The listing builds one solid part. Answer for the finished solid, in the listing's coordinates (mm). Coordinates: 2 decimals unless noted, no trailing zeros. Write each loop counter-clockwise with the first axis right and the second up, starting at its lowest first coordinate (ties: lowest second). Pieces come first, ordered by that corner, then holes. Notation, with made-up numbers: M 3,-12 L 62,-12 A15 cw 62,-6 Z; hole C -25.5,46.5 d7. An arc over 180 degrees is marked long. Put each result on its own line as item: value. Start each with the question number.
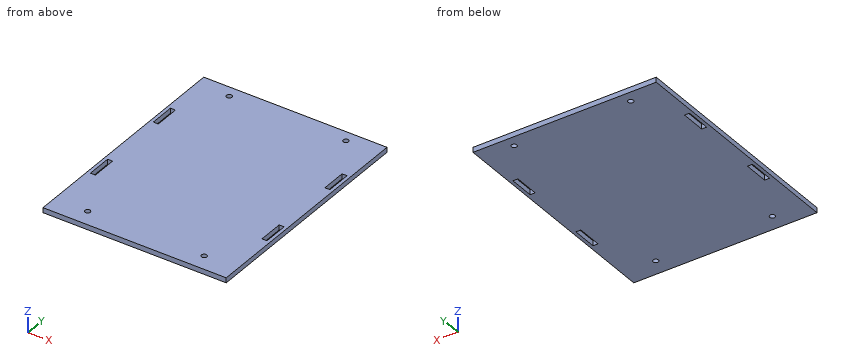
```python
from build123d import *

# Parameters (mm, degrees)
SKETCH_1_W      = 100
SKETCH_1_H      = 140.533333334
SKETCH_1_R      = 1.6
EXTRUDE_1_DEPTH = 3
EXTRUDE_2_DEPTH = 3


with BuildPart() as part:
    # 草图1 → 凸台-拉伸1 (new body)
    with BuildSketch(Plane.XY):
        with Locations((0, 54.4)):
            Rectangle(SKETCH_1_W, SKETCH_1_H)
        with Locations((-35, -6)):
            Circle(SKETCH_1_R, mode=Mode.SUBTRACT)
        with Locations((35, -6)):
            Circle(SKETCH_1_R, mode=Mode.SUBTRACT)
        with Locations((-35, 117.866666667)):
            Circle(SKETCH_1_R, mode=Mode.SUBTRACT)
        with Locations((35, 117.866666667)):
            Circle(SKETCH_1_R, mode=Mode.SUBTRACT)
    extrude(amount=-EXTRUDE_1_DEPTH)

    # 草图2 → 凸台-拉伸2 (add)
    with BuildSketch(Plane.XY):
        Polygon((-50, 92.666666667), (-50, 124.666666667), (-55, 124.666666667), (-55, -15.866666667), (-50, -15.866666667), (-50, 22.666666667), (-53, 22.666666667), (-53, 37.666666667), (-50, 37.666666667), (-50, 77.666666667), (-53, 77.666666667), (-53, 92.666666667), align=None)
    extrude_2 = extrude(amount=-EXTRUDE_2_DEPTH)

    # 镜向1: 凸台-拉伸2 across plane
    add(extrude_2.mirror(Plane(origin=(0, 0, 0), x_dir=(0, 0, 1), z_dir=(1, 0, 0))))


solid = part.part
```
1) A cutting plane is placed at A-A on y = -6. Write down the section's boundary in (x, z), then the cut area to 3 significant figures.
2) Straight lines are drawn through the part: probe 1 along X at (y, z) = (23, -0.9); probe 2 along Y at (x, z) = (-35, -1.1); probe 3 along X at (y, z) = (116.5, -0.1). For each, find the intervals that lie inside material, in ascending order.
3) Given pin 1 Ø3 at (x, y) = (35, 117.87) entering from +Z, flat-ended and moving along its own axis, determine where the tip first touches the part or whether it passes through.
4) A cutting plane is placed at B-B on x = 35. Write down the section's boundary in (y, z).
Answers follow:
1. outline: M -55,-3 L -36.6,-3 L -36.6,0 L -55,0 Z; M -33.4,-3 L 33.4,-3 L 33.4,0 L -33.4,0 Z; M 36.6,-3 L 55,-3 L 55,0 L 36.6,0 Z
1. area: 311 mm²
2. probe 1: x = -55 to -53, -50 to 50, 53 to 55
2. probe 2: y = -15.87 to -7.6, -4.4 to 116.27, 119.47 to 124.67
2. probe 3: x = -55 to -35.83, -34.17 to 34.17, 35.83 to 55
3. pin 1: passes through
4. outline: M -15.87,-3 L -7.6,-3 L -7.6,0 L -15.87,0 Z; M -4.4,-3 L 116.27,-3 L 116.27,0 L -4.4,0 Z; M 119.47,-3 L 124.67,-3 L 124.67,0 L 119.47,0 Z
